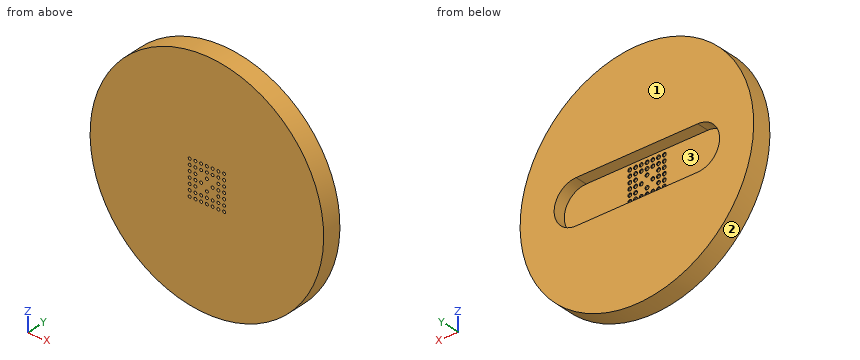
from build123d import *

# Parameters (mm, degrees)
SKETCH1_R                               = 60.96
BILLET_DEPTH                            = 10.16
KEROSENE_WELL_DEPTH                     = 6.35
FIRST_KEROSENE_OUTLET_REACH             = 88.807
SKETCH4_R                               = 0.7493
BOTTOM_NEEDLE_CHAMFER_SIZE              = 0.254
LPATTERN1_COUNT                         = 7
LPATTERN1_PITCH                         = 2.9972
LPATTERN1_COUNT_DIR2                    = 7
LPATTERN1_PITCH_DIR2                    = 2.9972
BOTTOM_NEEDLE_CHAMFER_OF_LPATTERN1_SIZE = 0.254


with BuildPart() as part:
    # Sketch1 → Billet (new body)
    with BuildSketch(Plane(origin=(0, 0, 0), x_dir=(1, 0, 0), z_dir=(0, 1, 0))):
        with Locations(Location((0, 0, 0), (0, 0, 270))):
            Circle(SKETCH1_R)
    extrude(amount=-BILLET_DEPTH)

    # Sketch2 → Kerosene Well (cut)
    with BuildSketch(Plane(origin=(0, 0, 0), x_dir=(1, 0, 0), z_dir=(0, 1, 0))):
        with BuildLine():
            Line((-31.75, 11.43), (31.75, 11.43))
            ThreePointArc((31.75, 11.43), (43.18, 0), (31.75, -11.43))
            Line((31.75, -11.43), (-31.75, -11.43))
            ThreePointArc((-31.75, -11.43), (-43.18, 0), (-31.75, 11.43))
        make_face()
    extrude(amount=-KEROSENE_WELL_DEPTH, mode=Mode.SUBTRACT)

    # Sketch4 → First Kerosene Outlet (cut, up to next)
    with BuildSketch(Plane(origin=(0, -10.16, 0), x_dir=(1, 0, 0), z_dir=(0, 1, 0)), mode=Mode.PRIVATE) as first_kerosene_outlet_sk1:
        with Locations(Location((8.9916, 8.9916, 0), (0, 0, 90))):
            Circle(SKETCH4_R)
    first_kerosene_outlet_tool1 = extrude(first_kerosene_outlet_sk1.sketch, amount=FIRST_KEROSENE_OUTLET_REACH, mode=Mode.PRIVATE) & part.part
    first_kerosene_outlet = first_kerosene_outlet_tool1.solids().sort_by_distance((8.9916, -10.16, -8.9916))[0]
    add(first_kerosene_outlet, mode=Mode.SUBTRACT)

    # Bottom Needle Chamfer
    bottom_needle_chamfer_edges = [part.edges().sort_by_distance(p)[0] for p in [
        (8.9916, -6.35, -8.2423),
    ]]
    chamfer(bottom_needle_chamfer_edges, length=BOTTOM_NEEDLE_CHAMFER_SIZE)

    # LPattern1: First Kerosene Outlet 7 × 7, 5 skipped
    with Locations(*[(-j * LPATTERN1_PITCH_DIR2, 0, i * LPATTERN1_PITCH) for i in range(LPATTERN1_COUNT) for j in range(LPATTERN1_COUNT_DIR2) if (i, j) not in ((0, 0), (2, 2), (2, 4), (3, 3), (4, 2), (4, 4))]):
        add(first_kerosene_outlet, mode=Mode.SUBTRACT)

    # Bottom Needle Chamfer of LPattern1
    bottom_needle_chamfer_of_lpattern1_edges = [part.edges().sort_by_distance(p)[0] for p in [
        (5.9944, -6.35, -8.2423),
        (2.9972, -6.35, -8.2423),
        (0, -6.35, -8.2423),
        (-2.9972, -6.35, -8.2423),
        (-5.9944, -6.35, -8.2423),
        (-8.9916, -6.35, -8.2423),
        (8.9916, -6.35, -5.2451),
        (5.9944, -6.35, -5.2451),
        (2.9972, -6.35, -5.2451),
        (0, -6.35, -5.2451),
        (-2.9972, -6.35, -5.2451),
        (-5.9944, -6.35, -5.2451),
        (-8.9916, -6.35, -5.2451),
        (8.9916, -6.35, -2.2479),
        (5.9944, -6.35, -2.2479),
        (0, -6.35, -2.2479),
        (-5.9944, -6.35, -2.2479),
        (-8.9916, -6.35, -2.2479),
        (8.9916, -6.35, 0.7493),
        (5.9944, -6.35, 0.7493),
        (2.9972, -6.35, 0.7493),
        (-2.9972, -6.35, 0.7493),
        (-5.9944, -6.35, 0.7493),
        (-8.9916, -6.35, 0.7493),
        (8.9916, -6.35, 3.7465),
        (5.9944, -6.35, 3.7465),
        (0, -6.35, 3.7465),
        (-5.9944, -6.35, 3.7465),
        (-8.9916, -6.35, 3.7465),
        (8.9916, -6.35, 6.7437),
        (5.9944, -6.35, 6.7437),
        (2.9972, -6.35, 6.7437),
        (0, -6.35, 6.7437),
        (-2.9972, -6.35, 6.7437),
        (-5.9944, -6.35, 6.7437),
        (-8.9916, -6.35, 6.7437),
        (8.9916, -6.35, 9.7409),
        (5.9944, -6.35, 9.7409),
        (2.9972, -6.35, 9.7409),
        (0, -6.35, 9.7409),
        (-2.9972, -6.35, 9.7409),
        (-5.9944, -6.35, 9.7409),
        (-8.9916, -6.35, 9.7409),
    ]]
    chamfer(bottom_needle_chamfer_of_lpattern1_edges, length=BOTTOM_NEEDLE_CHAMFER_OF_LPATTERN1_SIZE)


solid = part.part
The listing builds one solid part. Answer for the finished solid, in the listing's coordinates (mm). Face numbers are marked on the shaded views. Round coordinates to 2 decimals unless told otherwise and drop trailing zeros. Write each loop counter-clockwise with the first axis right and the second up, starting at its lowest first coordinate (ties: lowest second). Pieces come first, ordered by that corner, then holes. Notation, with made-up numbers: (37, 35.5) - (43, 35.5) arc R27 ccw to (43, 55.5) - close; hole circle Ø11 at (-1, 61). An arc over 180 degrees is marked (long way). Use a Markdown table: item, result. Add a question column.
1. The part is cut by section B-B (z = -28). Write down the section's boundary in (x, y), and give its area (3 significant figures).
2. The part is cut by section D-D (x = -21.5). Write down the section's boundary in (y, z), and give its area (3 significant figures).
3. The part is cut by section C-C (y = -8.5). Give the number of separate pieces and of enclosed holes in the cut face, and give its area (3 significant figures).
4. The part is cut by section A-A (x = 17.5). Write down the section's boundary in (y, z).
5. Consider line 1 (Z direction, x = 20, y = -2); line 2 (Z direction, x = 26.5, y = -1); line 3 (X direction, y = -3.75, z = 7.5). Determine where each line is inside the solid, lowest interval first.
6. Flat-ended cylindrical pins translate along their axes: P1, Ø1.9, axis at x = 8.99, z = 5.99, coming from the -Y side; P2, Ø1, axis at x = -42, y = -5.5, coming from the +Z side; P3, Ø1.7, axis at x = 0, z = -8.99, coming from the +Y side; P4, Ø2.5, axis at x = 0, z = 5.99, coming from the +Y side. Find the tip coordinate at first contact, or state that the pin passes through.
7. For a pull along X with two mould halves and no side action, classify the marked faces 1, 2 and 3 as +X half, -X half, draft (parallel to the pull), parting line (faces both ways), or undercut.
Reported:
| question | item | result |
|---|---|---|
| 1 | outline | (-54.15, -10.16) - (54.15, -10.16) - (54.15, 0) - (-54.15, 0) - close |
| 1 | area | 1,100 mm^2 |
| 2 | outline | (-10.16, -57.04) - (0, -57.04) - (0, -11.43) - (-6.35, -11.43) - (-6.35, 11.43) - (0, 11.43) - (0, 57.04) - (-10.16, 57.04) - close |
| 2 | area | 1,010 mm^2 |
| 3 | separate pieces | 1 |
| 3 | enclosed holes | 44 |
| 3 | area | 11,600 mm^2 |
| 4 | outline | (-10.16, -58.39) - (0, -58.39) - (0, -11.43) - (-6.35, -11.43) - (-6.35, 11.43) - (0, 11.43) - (0, 58.39) - (-10.16, 58.39) - close |
| 5 | line 1 | -57.59 to -11.43, 11.43 to 57.59 |
| 5 | line 2 | -54.9 to -11.43, 11.43 to 54.9 |
| 5 | line 3 | -60.5 to -40.38, 40.38 to 60.5 |
| 6 | P1 | y = -10.16 |
| 6 | P2 | z = 44.65 |
| 6 | P3 | y = -6.5 |
| 6 | P4 | y = -6.35 |
| 7 | face 1 | draft |
| 7 | face 2 | parting line |
| 7 | face 3 | undercut |
